The model under review builds one solid part; all positions refer to its coordinate system, in mm. Face numbers are marked on the shaded views. A direction names the side the tool comes from. Give positions to 0.01 mm unless a question says otherwise; leave off trailing zeros. Order: outer loops, then holes, each group sorted by start corner. A loop starts at its lowest first (then second) coordinate and runs counter-clockwise, first axis right, second up. Notation, with made-up numbers: (-18.5, -34.5) - (34.5, -34.5) arc R20 ccw to (34.5, -25.5) - close; hole circle Ø1 at (59, 5.25). An arc over 180 degrees is marked (long way). Write item = value, one per line. Start each with the question number.
1. We need section D-D, the plane x = -13. Give the boundary of the cut face in (y, z).
2. Mouldability with a two-part tool opening along X and no side actions: class the marked faces 4 and 5 as pulls with the +X half, pulls with the -X half, needs draft (parallel to the pull), parting line crosses it, or undercut.
3. Machinability: for the marked faces 1, 2 and 3, which of the approach directions +Z, -Z, +X, -X, +Y, -Y give a long, thin tool a straight path to every point of the face, cutting with its end or side? Answer none if there is none.
4. We need section C-C, the plane x = 6.5. Give the boundary of the cut face in (y, z).
5. For P1, Ø3.5, axis at x = -38.5, z = 0, coming from the -Y side; P2, Ø2, axis at x = -2, y = -98, coming from the +Z side; P3, Ø2, axis at x = -0.5, z = 1.5, coming from the -Y side, all flat-tipped, find the tip position at first contact; note any pin that passes through.
6. We need section A-A, the plane z = 9.25. State how many separate pieces and enclosed holes the cut face has, and give its area (3 significant figures).
7. Wall thickness on probe 1 along X at (y, z) = (-101, -1); probe 2 along X at (y, z) = (-114, 2); probe 3 along Y at (x, z) = (2, 14): over which ranges is each line inside the solid? List them lowest first.
8. We need section B-B, the plane y = -183.5. Give the boundary of the cut face in (x, z).
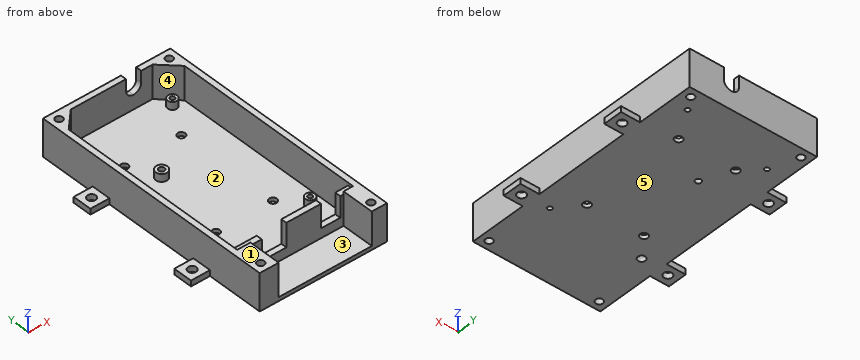
from build123d import *

# Parameters (mm, degrees)
SKETCH1_W           = 67
SKETCH1_H           = 130
BOSS_EXTRUDE1_DEPTH = 2
SKETCH2_W           = 18.2532
SKETCH2_H           = 3
BOSS_EXTRUDE2_DEPTH = 17.5
SKETCH3_R           = 3
SKETCH3_R_2         = 1.5
SKETCH3_R_3         = 2.5
SKETCH3_R_4         = 1.2
SKETCH3_R_5         = 4
SKETCH3_R_6         = 2
BOSS_EXTRUDE3_DEPTH = 4
SKETCH4_W           = 12.938
SKETCH4_H           = 3
SKETCH4_W_2         = 10.144
BOSS_EXTRUDE4_DEPTH = 5
SKETCH5_R           = 2
CUT_EXTRUDE1_DEPTH  = 201.297076365
SKETCH6_W           = 12.940950003
SKETCH6_H           = 3
CUT_EXTRUDE2_DEPTH  = 1.5
SKETCH7_W           = 10
SKETCH7_H           = 16.939031541
SKETCH7_W_2         = 8
BOSS_EXTRUDE5_DEPTH = 17.5
SKETCH8_W           = 6.723849997
SKETCH8_H           = 3
CUT_EXTRUDE3_DEPTH  = 1.5
CHAMFER1_SIZE       = 9
SKETCH10_R          = 1.9
CUT_EXTRUDE4_DEPTH  = 201.481716873
SKETCH11_R          = 2
CUT_EXTRUDE5_DEPTH  = 201.297076365
SKETCH13_W          = 8
SKETCH13_H          = 3
CUT_EXTRUDE6_DEPTH  = 10
FILLET1_R           = 4
SKETCH14_W          = 10
SKETCH14_H          = 10
SKETCH14_R          = 2.2
BOSS_EXTRUDE6_DEPTH = 3
SKETCH15_R          = 1.2
SKETCH15_R_2        = 1.5
CUT_EXTRUDE7_DEPTH  = 203.281693166


with BuildPart() as part:
    # Sketch1 → Boss-Extrude1 (new body)
    with BuildSketch(Plane.XY):
        with Locations((1.448229487, -131.44665957)):
            Rectangle(SKETCH1_W, SKETCH1_H)
    extrude(amount=-BOSS_EXTRUDE1_DEPTH)

    # Sketch2 → Boss-Extrude2 (add)
    with BuildSketch(Plane.XY):
        Polygon((-32.051770513, -66.44665957), (34.948229487, -66.44665957), (34.948229487, -179.507628029), (25.22437949, -179.507628029), (25.22437949, -176.507628029), (31.948229487, -176.507628029), (31.948229487, -69.44665957), (-29.051770513, -69.44665957), (-29.051770513, -176.507628029), (-16.11082051, -176.507628029), (-16.11082051, -179.507628029), (-32.051770513, -179.507628029), align=None)
        with Locations((5.95377949, -178.007628029)):
            Rectangle(SKETCH2_W, SKETCH2_H)
    extrude(amount=BOSS_EXTRUDE2_DEPTH)

    # Sketch3 → Boss-Extrude3 (add)
    # profile 1 of 5: a face of its own
    with BuildSketch(Plane.XY):
        with Locations(Location((-6.90031328, -108.930928029, 0), (0, 0, 180))):
            Circle(SKETCH3_R)
        with Locations(Location((-6.90031328, -108.930928029, 0), (0, 0, 180))):
            Circle(SKETCH3_R_2, mode=Mode.SUBTRACT)
    # profile 2 of 5: a face of its own
    with BuildSketch(Plane.XY):
        with Locations(Location((-22.341820513, -85.423228029, 0), (0, 0, 180))):
            Circle(SKETCH3_R_3)
        with Locations(Location((-22.341820513, -85.423228029, 0), (0, 0, 180))):
            Circle(SKETCH3_R_4, mode=Mode.SUBTRACT)
    # profile 3 of 5: a face of its own
    with BuildSketch(Plane.XY):
        with Locations(Location((25.994379487, -77.930228029, 0), (0, 0, 180))):
            Circle(SKETCH3_R_3)
        with Locations(Location((25.994379487, -77.930228029, 0), (0, 0, 180))):
            Circle(SKETCH3_R_4, mode=Mode.SUBTRACT)
    # profile 4 of 5: a face of its own
    with BuildSketch(Plane.XY):
        with Locations(Location((25.994379487, -160.556428029, 0), (0, 0, 180))):
            Circle(SKETCH3_R_3)
        with Locations(Location((25.994379487, -160.556428029, 0), (0, 0, 180))):
            Circle(SKETCH3_R_4, mode=Mode.SUBTRACT)
    # profile 5 of 5: a face of its own
    with BuildSketch(Plane.XY):
        with Locations(Location((-22.341820513, -160.556428029, 0), (0, 0, 180))):
            Circle(SKETCH3_R_5)
        with Locations(Location((-22.341820513, -160.556428029, 0), (0, 0, 180))):
            Circle(SKETCH3_R_6, mode=Mode.SUBTRACT)
    extrude(amount=BOSS_EXTRUDE3_DEPTH)

    # Sketch4 → Boss-Extrude4 (add)
    with BuildSketch(Plane.XY):
        with Locations((-9.64182051, -178.007628029)):
            Rectangle(SKETCH4_W, SKETCH4_H)
        with Locations((20.15237949, -178.007628029)):
            Rectangle(SKETCH4_W_2, SKETCH4_H)
    extrude(amount=BOSS_EXTRUDE4_DEPTH)

    # Sketch5 → Cut-Extrude1 (cut, through all)
    with BuildSketch(Plane.XY):
        with Locations((-13.551770513, -94.136094707)):
            Circle(SKETCH5_R)
        with Locations((16.448229487, -94.136094707)):
            Circle(SKETCH5_R)
        with Locations((-13.551770513, -149.136094707)):
            Circle(SKETCH5_R)
        with Locations((16.448229487, -149.136094707)):
            Circle(SKETCH5_R)
    extrude(amount=-CUT_EXTRUDE1_DEPTH, mode=Mode.SUBTRACT)

    # Sketch6 → Cut-Extrude2 (cut)
    with BuildSketch(Plane.XY.offset(17.5)):
        with Locations((-22.581295512, -178.007628029)):
            Rectangle(SKETCH6_W, SKETCH6_H)
    extrude(amount=-CUT_EXTRUDE2_DEPTH, mode=Mode.SUBTRACT)

    # Sketch7 → Boss-Extrude5 (add)
    with BuildSketch(Plane.XY):
        with Locations((-27.051770513, -187.9771438)):
            Rectangle(SKETCH7_W, SKETCH7_H)
        with Locations((30.948229487, -187.9771438)):
            Rectangle(SKETCH7_W_2, SKETCH7_H)
    extrude(amount=BOSS_EXTRUDE5_DEPTH)

    # Sketch8 → Cut-Extrude3 (cut)
    with BuildSketch(Plane.XY.offset(17.5)):
        with Locations((28.586304489, -178.007628029)):
            Rectangle(SKETCH8_W, SKETCH8_H)
    extrude(amount=-CUT_EXTRUDE3_DEPTH, mode=Mode.SUBTRACT)

    # Chamfer1
    chamfer1_edges = [part.edges().sort_by_distance(p)[0] for p in [
        (-29.051770513, -69.44665957, 8.75),
        (31.948229487, -69.44665957, 8.75),
    ]]
    chamfer(chamfer1_edges, length=CHAMFER1_SIZE)

    # Sketch10 → Cut-Extrude4 (cut, through all)
    with BuildSketch(Plane.XY.offset(17.5)):
        with Locations((-27.551770513, -70.94665957)):
            Circle(SKETCH10_R)
        with Locations(Location((30.448229487, -70.94665957, 0), (0, 0, 180))):
            Circle(SKETCH10_R)
        with Locations((-27.551770513, -191.94665957)):
            Circle(SKETCH10_R)
        with Locations((30.448229487, -191.94665957)):
            Circle(SKETCH10_R)
    extrude(amount=-CUT_EXTRUDE4_DEPTH, mode=Mode.SUBTRACT)

    # Sketch11 → Cut-Extrude5 (cut, through all)
    with BuildSketch(Plane.XY):
        with Locations(Location((-22.341820513, -160.556428029, 0), (0, 0, 180))):
            Circle(SKETCH11_R)
    extrude(amount=-CUT_EXTRUDE5_DEPTH, mode=Mode.SUBTRACT)

    # Sketch13 → Cut-Extrude6 (cut)
    with BuildSketch(Plane.XY.offset(17.5)):
        with Locations((13.007373808, -67.94665957)):
            Rectangle(SKETCH13_W, SKETCH13_H)
    extrude(amount=-CUT_EXTRUDE6_DEPTH, mode=Mode.SUBTRACT)

    # Fillet1
    fillet1_edges = [part.edges().sort_by_distance(p)[0] for p in [
        (17.007373808, -67.94665957, 7.5),
        (9.007373808, -67.94665957, 7.5),
    ]]
    fillet(fillet1_edges, radius=FILLET1_R - 0.0001)  # a hair under: the kernel refuses the full size

    # Sketch14 → Boss-Extrude6 (add)
    # profile 1 of 4: a face of its own
    with BuildSketch(Plane(origin=(0, 0, -2), x_dir=(-1, 0, 0), z_dir=(0, 0, -1))):
        with Locations((37.051770513, -101.268546353)):
            Rectangle(SKETCH14_W, SKETCH14_H)
        with Locations((37.051770513, -101.268546353)):
            Circle(SKETCH14_R, mode=Mode.SUBTRACT)
    # profile 2 of 4: a face of its own
    with BuildSketch(Plane(origin=(0, 0, -2), x_dir=(-1, 0, 0), z_dir=(0, 0, -1))):
        with Locations((-39.948229487, -101.268546353)):
            Rectangle(SKETCH14_W, SKETCH14_H)
        with Locations(Location((-39.948229487, -101.268546353, 0), (0, 0, 180))):
            Circle(SKETCH14_R, mode=Mode.SUBTRACT)
    # profile 3 of 4: a face of its own
    with BuildSketch(Plane(origin=(0, 0, -2), x_dir=(-1, 0, 0), z_dir=(0, 0, -1))):
        with Locations((-39.948229487, -161.624772787)):
            Rectangle(SKETCH14_W, SKETCH14_H)
        with Locations((-39.948229487, -161.624772787)):
            Circle(SKETCH14_R, mode=Mode.SUBTRACT)
    # profile 4 of 4: a face of its own
    with BuildSketch(Plane(origin=(0, 0, -2), x_dir=(-1, 0, 0), z_dir=(0, 0, -1))):
        with Locations((37.051770513, -161.624772787)):
            Rectangle(SKETCH14_W, SKETCH14_H)
        with Locations(Location((37.051770513, -161.624772787, 0), (0, 0, 180))):
            Circle(SKETCH14_R, mode=Mode.SUBTRACT)
    extrude(amount=-BOSS_EXTRUDE6_DEPTH)

    # Sketch15 → Cut-Extrude7 (cut, through all)
    with BuildSketch(Plane.XY):
        with Locations(Location((-22.341820513, -85.423228029, 0), (0, 0, 180))):
            Circle(SKETCH15_R)
        with Locations(Location((25.994379487, -77.930228029, 0), (0, 0, 180))):
            Circle(SKETCH15_R)
        with Locations(Location((-6.90031328, -108.930928029, 0), (0, 0, 180))):
            Circle(SKETCH15_R_2)
        with Locations(Location((25.994379487, -160.556428029, 0), (0, 0, 180))):
            Circle(SKETCH15_R)
    extrude(amount=-CUT_EXTRUDE7_DEPTH, mode=Mode.SUBTRACT)


solid = part.part
Model answer:
q1.outline = (-196.45, -2) - (-151.06, -2) - (-151.06, 0) - (-176.51, 0) - (-176.51, 5) - (-179.51, 5) - (-179.51, 0) - (-196.45, 0) - close; (-147.21, -2) - (-96.06, -2) - (-96.06, 0) - (-147.21, 0) - close; (-92.21, -2) - (-66.45, -2) - (-66.45, 17.5) - (-69.45, 17.5) - (-69.45, 0) - (-92.21, 0) - close
q2.face_4 = undercut
q2.face_5 = needs draft
q3.face_1 = +Z, +X, -X, +Y, -Y
q3.face_2 = +Z
q3.face_3 = +Z, -Y
q4.outline = (-196.45, -2) - (-66.45, -2) - (-66.45, 17.5) - (-69.45, 17.5) - (-69.45, 0) - (-176.51, 0) - (-176.51, 17.5) - (-179.51, 17.5) - (-179.51, 0) - (-196.45, 0) - close
q5.P1 = -166.62
q5.P2 = 0
q5.P3 = -179.51
q6.separate_pieces = 3
q6.enclosed_holes = 4
q6.area = 1,300 mm2
q7.probe_1 = -42.05 to -39.24, -34.87 to 37.76, 42.13 to 44.95
q7.probe_2 = -32.05 to -29.05, 31.95 to 34.95
q7.probe_3 = -179.51 to -176.51, -69.45 to -66.45
q8.outline = (-32.05, -2) - (34.95, -2) - (34.95, 17.5) - (26.95, 17.5) - (26.95, 0) - (-22.05, 0) - (-22.05, 17.5) - (-32.05, 17.5) - close
